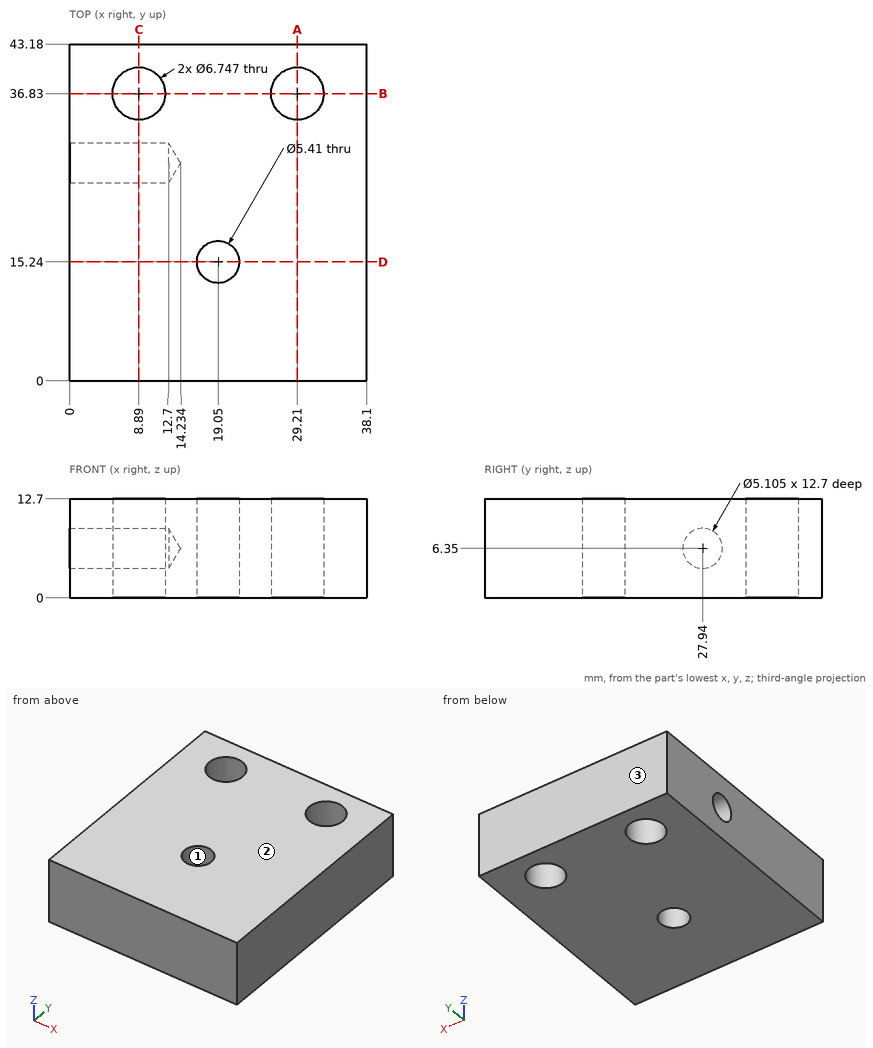
Design review of the part shown in the three views and the two pictorial views. Dimensions are in mm from the part's minimum x, y and z. Give positions to 0.01 mm unless a question says otherwise; leave off trailing zeros. Order: outer loops, then holes, each group sorted by start corner. A loop starts at its lowest first (then second) coordinate and runs counter-clockwise, first axis right, second up. Notation, with made-up numbers: (56.25, 84) -> (69.25, 84) arc R26 cw to (69.25, 108) -> close; hole circle Ø4 at (-7, 11). An arc over 180 degrees is marked (long way). Write each question's results on one line, items separated by ' | '. Start each with the question number.
Q1. Add section B-B on y = 36.83. Give the boundary of the cut face in (x, z).
Q2. Add section C-C on x = 8.89. State how many separate pieces and enclosed holes the cut face has, and give its area (3 significant figures).
Q3. Mouldability with a two-part tool opening along Y and no side actions: class the marked faces 1, 2 and 3 as +Y half, -Y half, draft (parallel to the pull), parting line (faces both ways), or undercut.
Q4. Add section D-D on y = 15.24. Give the boundary of the cut face in (x, z) (1 decimal).
Q5. Wall thickness on L1, parallel to X at y = 37, z = 5.5; L2, parallel to Y at x = 29.21, z = 6; L3, parallel to Y at x = 19.05, z = 6.5 (1 decimal): over which ranges is each line inside the solid? List them lowest first. Write a range as from..to.
Q6. Add section A-A on x = 29.21. Give the boundary of the cut face in (y, z).
Found:
1) outline: (0, 0) -> (5.52, 0) -> (5.52, 12.7) -> (0, 12.7) -> close; (12.26, 0) -> (25.84, 0) -> (25.84, 12.7) -> (12.26, 12.7) -> close; (32.58, 0) -> (38.1, 0) -> (38.1, 12.7) -> (32.58, 12.7) -> close
2) separate pieces: 2 | enclosed holes: 1 | area: 442 mm2
3) face 1: undercut | face 2: draft | face 3: +Y half
4) outline: (0, 0) -> (16.3, 0) -> (16.3, 12.7) -> (0, 12.7) -> close; (21.8, 0) -> (38.1, 0) -> (38.1, 12.7) -> (21.8, 12.7) -> close
5) L1: x = 0..5.52, 12.26..25.84, 32.58..38.1 | L2: y = 0..33.46, 40.2..43.18 | L3: y = 0..12.5, 17.9..43.2
6) outline: (0, 0) -> (33.46, 0) -> (33.46, 12.7) -> (0, 12.7) -> close; (40.2, 0) -> (43.18, 0) -> (43.18, 12.7) -> (40.2, 12.7) -> close
